The listing builds one solid part. Answer for the finished solid, in the listing's coordinates (mm). A direction names the side the tool comes from. Round coordinates to 2 decimals unless told otherwise and drop trailing zeros. Loops run counter-clockwise (first coordinate to the right, second up) from the corner with the lowest first, then second, coordinate; pieces in that order, holes last. Notation, with made-up numbers: (-12, -14.5) -> (47, -14.5) arc R20 ccw to (47, -9.5) -> close; hole circle Ø1 at (89.5, -8.5). An arc over 180 degrees is marked (long way). Write each question's results on one line, items separated by ' | '. Start each with the question number.
(1) Straight lines are drawn through the part: probe 1 along Y at (x, z) = (-12.7, 890.25) (3 decimals); probe 2 along X at (y, z) = (1.75, 47.5); probe 3 along Y at (x, z) = (12.7, 893) (3 decimals). For each, find the intervals that lie inside material, in ascending order.
(2) The part is cut by section A-A (z = 400.5). Determine the outline of the cut face in (x, y) (3 decimals), plus the area to 3 significant figures.
(3) The part is cut by section B-B (y = -27.5). Determine the outline of the cut face in (x, z) (3 decimals).
(4) For faces 1 (the face through (0, 3.155, 454)), 2 (the face through (0, -49, 888.575)), determine the directions among +Z, -Z, +X, -X, +Y, -Y from which every point of the face is accessible in a straight line to the end or side of a thin tool.
(5) Determine the mould class of faces 3 (the face through (25.4, -2, 450)), 4 (the face through (0, -3.155, 451)), 5 (the face through (-25.4, 2, 450)) for opening direction X: released by +X, released by -X, zero draft, split by the parting line, or undercut.
(6) Flat-ended cylindrical pins translate along their axes: pin 1 (15 mm diameter, centred on x = 1, y = -46.5, fed in from -Z) (3 decimals); pin 2 (3 mm diameter, centred on x = -11, z = 585.5, fed in from -Y) (3 decimals). Find the tip coordinate at first contact, or state that the pin passes through.
```python
from build123d import *

# Parameters (mm, degrees)
CROQUIS1_W            = 50.8
CROQUIS1_H            = 6.31
CROQUIS2_R            = 6.5
CORTAR_EXTRUIR1_DEPTH = 10
CROQUIS3_R            = 6.5
CORTAR_EXTRUIR2_DEPTH = 10
CROQUIS4_W            = 59.2
CROQUIS4_H            = 50.8
CORTAR_EXTRUIR3_DEPTH = 10
CROQUIS5_R            = 5
CORTAR_EXTRUIR4_DEPTH = 10


with BuildPart() as part:
    # Barrer1: sweep along a curve in space
    with BuildLine() as barrer1_path:
        Line((0, 0, 0), (0, 0, 891.73))
        Line((0, 0, 891.73), (0, -67.38, 891.73))
        Line((0, -67.38, 891.73), (84.6, -67.38, 891.73))
    # Croquis1 → Barrer1 (sweep)
    with BuildSketch(Plane.XY):
        Rectangle(CROQUIS1_W, CROQUIS1_H)
    sweep(path=barrer1_path.line, transition=Transition.RIGHT)

    # Croquis2 → Cortar-Extruir1 (cut)
    with BuildSketch(Plane(origin=(0, 3.155, 0), x_dir=(1, 0, 0), z_dir=(0, 1, 0))):
        with Locations(Location((0, -16.5, 0), (0, 0, 270))):
            Circle(CROQUIS2_R)
        with Locations(Location((0, -47.5, 0), (0, 0, 270))):
            Circle(CROQUIS2_R)
    extrude(amount=-CORTAR_EXTRUIR1_DEPTH, mode=Mode.SUBTRACT)

    # Croquis3 → Cortar-Extruir2 (cut)
    with BuildSketch(Plane(origin=(0, 0, 888.575), x_dir=(-1, 0, 0), z_dir=(0, 0, -1))):
        with Locations((-60, -67.38)):
            Circle(CROQUIS3_R)
    extrude(amount=-CORTAR_EXTRUIR2_DEPTH, mode=Mode.SUBTRACT)

    # Croquis4 → Cortar-Extruir3 (cut)
    with BuildSketch(Plane.XY.offset(894.885)):
        with Locations((55, -67.38)):
            Rectangle(CROQUIS4_W, CROQUIS4_H)
    extrude(amount=-CORTAR_EXTRUIR3_DEPTH, mode=Mode.SUBTRACT)

    # Croquis5 → Cortar-Extruir4 (cut)
    with BuildSketch(Plane(origin=(0, 0, 888.575), x_dir=(-1, 0, 0), z_dir=(0, 0, -1))):
        with Locations(Location((-12.7, -54.68, 0), (0, 0, 315))):
            Circle(CROQUIS5_R)
        with Locations(Location((12.7, -80.08, 0), (0, 0, 315))):
            Circle(CROQUIS5_R)
    extrude(amount=-CORTAR_EXTRUIR4_DEPTH, mode=Mode.SUBTRACT)


solid = part.part
```
Checked values:
1) probe 1: y = -92.78 to -85.08, -75.08 to 3.155 | probe 2: x = -25.4 to -6.5, 6.5 to 25.4 | probe 3: y = -92.78 to -59.68, -49.68 to 3.155
2) outline: (-25.4, -3.155) -> (25.4, -3.155) -> (25.4, 3.155) -> (-25.4, 3.155) -> close | area: 321 mm2
3) outline: (-25.4, 888.575) -> (25.4, 888.575) -> (25.4, 894.885) -> (-25.4, 894.885) -> close
4) face 1: +Z, -Z, +X, -X, +Y | face 2: -Z, +X, -X, -Y
5) face 3: released by +X | face 4: zero draft | face 5: released by -X
6) pin 1: stops at z = 888.575 | pin 2: stops at y = -3.155
